```python
from build123d import *

# Parameters (mm, degrees)
SKETCH1_W           = 81.28
SKETCH1_H           = 12.7
BOSS_EXTRUDE1_DEPTH = 12.7
SKETCH2_W           = 69.20484
SKETCH2_H           = 12.7
BOSS_EXTRUDE2_DEPTH = 9.525
SKETCH3_R           = 1.25
CUT_EXTRUDE2_DEPTH  = 84.24072561
SKETCH5_R           = 3.556
CUT_EXTRUDE3_DEPTH  = 1.99898
SKETCH6_R           = 2.19964
CUT_EXTRUDE4_DEPTH  = 1.27
SKETCH7_R           = 1.650000002
CUT_EXTRUDE5_DEPTH  = 6.604


with BuildPart() as part:
    # Sketch1 → Boss-Extrude1 (new body)
    with BuildSketch(Plane(origin=(0, 0, 0), x_dir=(1, 0, 0), z_dir=(0, 1, 0))):
        with Locations((40.64, 6.35)):
            Rectangle(SKETCH1_W, SKETCH1_H)
    extrude(amount=BOSS_EXTRUDE1_DEPTH)

    # Sketch2 → Boss-Extrude2 (add)
    with BuildSketch(Plane(origin=(0, 12.7, 0), x_dir=(1, 0, 0), z_dir=(0, 1, 0))):
        with Locations((40.64, 6.35)):
            Rectangle(SKETCH2_W, SKETCH2_H)
    extrude(amount=BOSS_EXTRUDE2_DEPTH)

    # Sketch3 → Cut-Extrude2 (cut, through all)
    with BuildSketch(Plane(origin=(0, 12.7, 0), x_dir=(1, 0, 0), z_dir=(0, 1, 0))):
        with Locations(Location((3.01879, 6.35, 0), (0, 0, 270))):
            Circle(SKETCH3_R)
        with Locations(Location((78.26121, 6.35, 0), (0, 0, 270))):
            Circle(SKETCH3_R)
    extrude(amount=-CUT_EXTRUDE2_DEPTH, mode=Mode.SUBTRACT)

    # Sketch5 → Cut-Extrude3 (cut)
    with BuildSketch(Plane.XZ):
        with Locations((3.01879, -6.35)):
            Circle(SKETCH5_R)
        with Locations((78.26121, -6.35)):
            Circle(SKETCH5_R)
    extrude(amount=-CUT_EXTRUDE3_DEPTH, mode=Mode.SUBTRACT)

    # Sketch6 → Cut-Extrude4 (cut)
    with BuildSketch(Plane(origin=(0, 0, -12.7), x_dir=(-1, 0, 0), z_dir=(0, 0, -1))):
        with Locations((-40.64, 13.29944)):
            Circle(SKETCH6_R)
    extrude(amount=-CUT_EXTRUDE4_DEPTH, mode=Mode.SUBTRACT)

    # Sketch7 → Cut-Extrude5 (cut)
    with BuildSketch(Plane(origin=(0, 0, -11.43), x_dir=(-1, 0, 0), z_dir=(0, 0, -1))):
        with Locations((-40.64, 13.29944)):
            Circle(SKETCH7_R)
    extrude(amount=-CUT_EXTRUDE5_DEPTH, mode=Mode.SUBTRACT)


solid = part.part
```
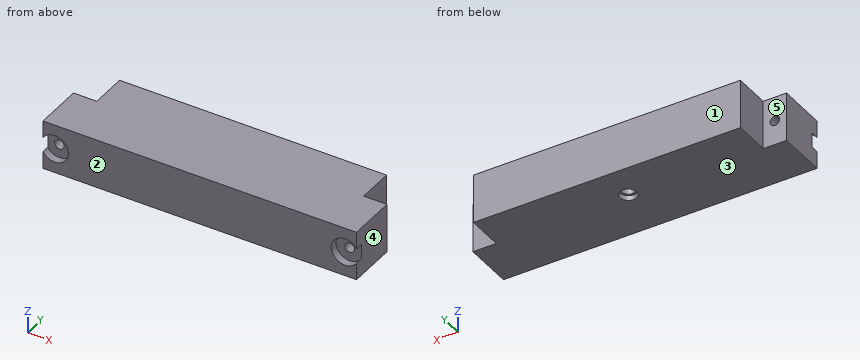
For this review, take the finished solid that the model builds, in its own axes (mm). Face numbers are marked on the shaded views. A direction names the side the tool comes from. Round coordinates to 2 decimals unless told otherwise and drop trailing zeros. Write each loop counter-clockwise with the first axis right and the second up, starting at its lowest first coordinate (ties: lowest second). Pieces come first, ordered by that corner, then holes.
1) Insertion check: pin 1 Ø1 at (x, y) = (40, 13.5) entering from -Z; pin 2 Ø5 at (x, z) = (3.5, -9.5) entering from +Y; pin 3 Ø2 at (x, z) = (3.02, -6.35) entering from -Y; pin 4 Ø2 at (x, z) = (4.5, -8) entering from -Y. Each pin has a flat end and moves straight along its axis. Give the tip position at first contact, or say it passes through.
Answer below:
pin 1: stops at z = -4.83
pin 2: stops at y = 12.7
pin 3: passes through
pin 4: stops at y = 2
2) For line 1 along X through (y, z) = (7.75, -6.35); line 2 along Y through (x, z) = (40.64, -7) (3 decimals); line 3 along X through (y, z) = (10, -5.25), list the stretches that pass through material, from the lowest coordinate up.
Answer below:
line 1: x = 0 to 1.77, 4.27 to 77.01, 79.51 to 81.28
line 2: y = 0 to 11.649, 14.949 to 22.225
line 3: x = 0 to 2.43, 3.61 to 77.67, 78.85 to 81.28
3) Mouldability with a two-part tool opening along Y and no side actions: class the marked faces 1, 2 and 3 as +Y half, -Y half, draft (parallel to the pull), parting line (faces both ways), or undercut.
Answer below:
face 1: +Y half
face 2: -Y half
face 3: draft
4) Machinability: for the marked faces 4 and 5, which of the approach directions +Z, -Z, +X, -X, +Y, -Y give a long, thin tool a straight path to every point of the face, cutting with its end or side? Answer none if there is none.
Answer below:
face 4: +Z, -Z, +X, +Y, -Y
face 5: +Z, -Z, -X, +Y
5) Take a section at B-B on x = 40.64. Give the boundary of the cut face in (y, z) (3 decimals), then the cut area to 3 significant figures.
Answer below:
outline: (0, -12.7) - (11.1, -12.7) - (11.1, -11.43) - (11.649, -11.43) - (11.649, -4.826) - (14.949, -4.826) - (14.949, -11.43) - (15.499, -11.43) - (15.499, -12.7) - (22.225, -12.7) - (22.225, 0) - (0, 0) - close
area: 255 mm2
6) Take a section at C-C on y = 20.5. Give the boundary of the cut face in (x, z), then the cut area to 3 significant figures.
Answer below:
outline: (6.04, -12.7) - (75.24, -12.7) - (75.24, 0) - (6.04, 0) - close
area: 879 mm2
7) Take a section at A-A on z = -6.35. Give the boundary of the cut face in (x, y) (3 decimals), then the cut area to 3 significant figures.
Answer below:
outline: (0, 1.999) - (1.769, 1.999) - (1.769, 12.7) - (0, 12.7) - close; (4.269, 1.999) - (6.575, 1.999) - (6.575, 0) - (74.705, 0) - (74.705, 1.999) - (77.011, 1.999) - (77.011, 12.7) - (75.242, 12.7) - (75.242, 22.225) - (6.038, 22.225) - (6.038, 12.7) - (4.269, 12.7) - close; (79.511, 1.999) - (81.28, 1.999) - (81.28, 12.7) - (79.511, 12.7) - close; hole circle Ø3.3 at (40.64, 13.299)
area: 1,600 mm2
